Verification items for this drawing (mm, ordinates from the low corner). A direction names the side the tool comes from. Coordinates: 2 decimals unless noted, no trailing zeros. Loops run counter-clockwise (first coordinate to the right, second up) from the corner with the lowest first, then second, coordinate; pieces in that order, holes last. Notation, with made-up numbers: M -28.5,40.5 L -16.5,40.5 A20 cw -16.5,71.5 Z; hole C 11,1 d2. An arc over 180 degrees is marked long. Return JSON: item names as keys, results as strings.
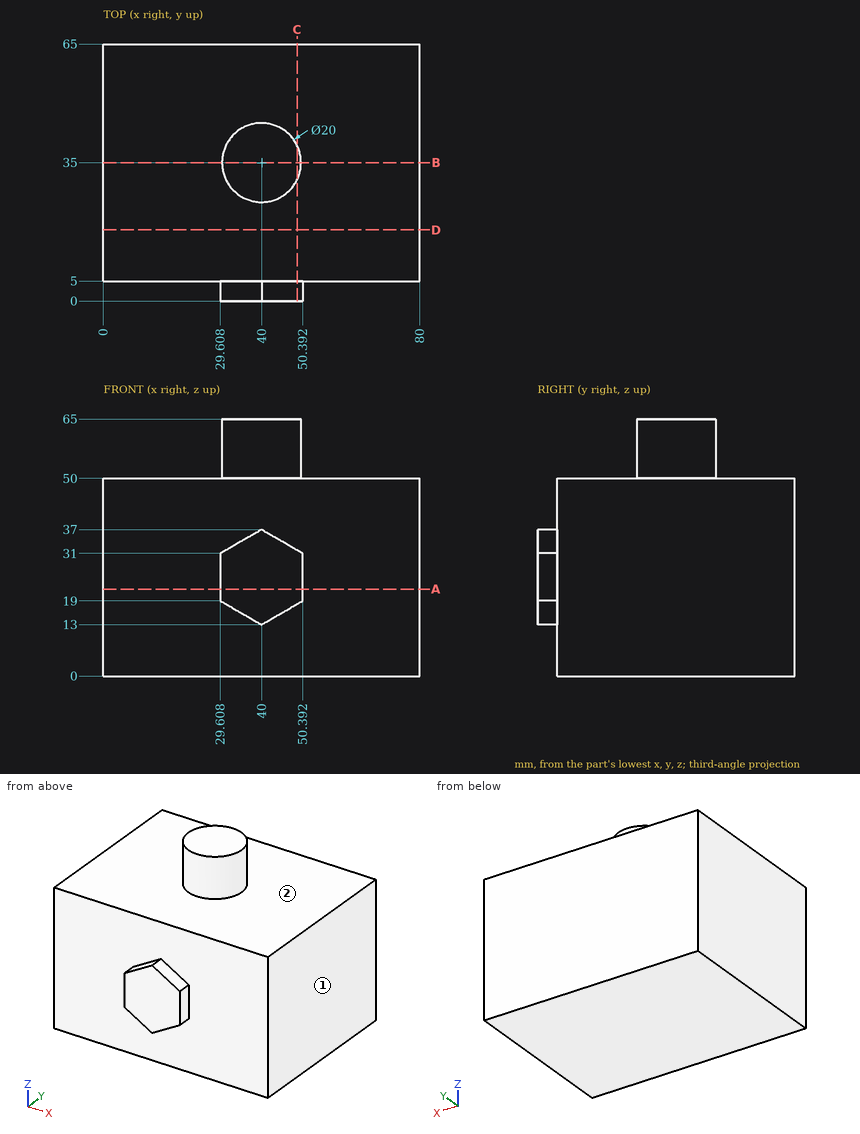
1) Scan lines: line 1 along Z through (x, y) = (59, 17); line 2 along Y through (x, z) = (11, 4); line 3 along Y through (x, z) = (34, 57). Record each from-to range of solid material in increasing order. Write a range as [from, to].
Answers:
{"line 1": "[0, 50]", "line 2": "[5, 65]", "line 3": "[27, 43]"}
2) Go/stop test with flat-tipped pins: pin 1 Ø12 at (x, z) = (16.5, 13.5) entering from -Y; pin 2 Ø6 at (y, z) = (14, 19) entering from -X; pin 3 Ø4 at (x, y) = (36.5, 16.5) entering from +Z; pin 4 Ø4 at (y, z) = (2, 27) entering from -X. Record where each tip stops, or that it passes through.
Answers:
{"pin 1": "y = 5", "pin 2": "x = 0", "pin 3": "z = 50", "pin 4": "x = 29.61"}
3) Set-up check for the marked faces 1 and 2: record each of +Z, -Z, +X, -X, +Y, -Y from which the full face is reachable in a straight line by a thin tool's end or side.
Answers:
{"face 1": "+Z, -Z, +X, +Y, -Y", "face 2": "+Z"}
4) Section check B-B on y = 35. Record the cut outline in (x, z), then the cut area to 3 significant figures.
Answers:
{"outline": "M 0,0 L 80,0 L 80,50 L 50,50 L 50,65 L 30,65 L 30,50 L 0,50 Z", "area": "4,300 mm²"}
5) Section check C-C on x = 49. Record the cut outline in (y, z).
Answers:
{"outline": "M 0,18.2 L 5,18.2 L 5,0 L 65,0 L 65,50 L 39.36,50 L 39.36,65 L 30.64,65 L 30.64,50 L 5,50 L 5,31.8 L 0,31.8 Z"}
6) Section check A-A on z = 22. Record the cut outline in (x, y), then the cut area to 3 significant figures.
Answers:
{"outline": "M 0,5 L 29.61,5 L 29.61,0 L 50.39,0 L 50.39,5 L 80,5 L 80,65 L 0,65 Z", "area": "4,900 mm²"}
7) Section check D-D on y = 18. Record the cut outline in (x, z), then the cut area to 3 significant figures.
Answers:
{"outline": "M 0,0 L 80,0 L 80,50 L 0,50 Z", "area": "4,000 mm²"}
